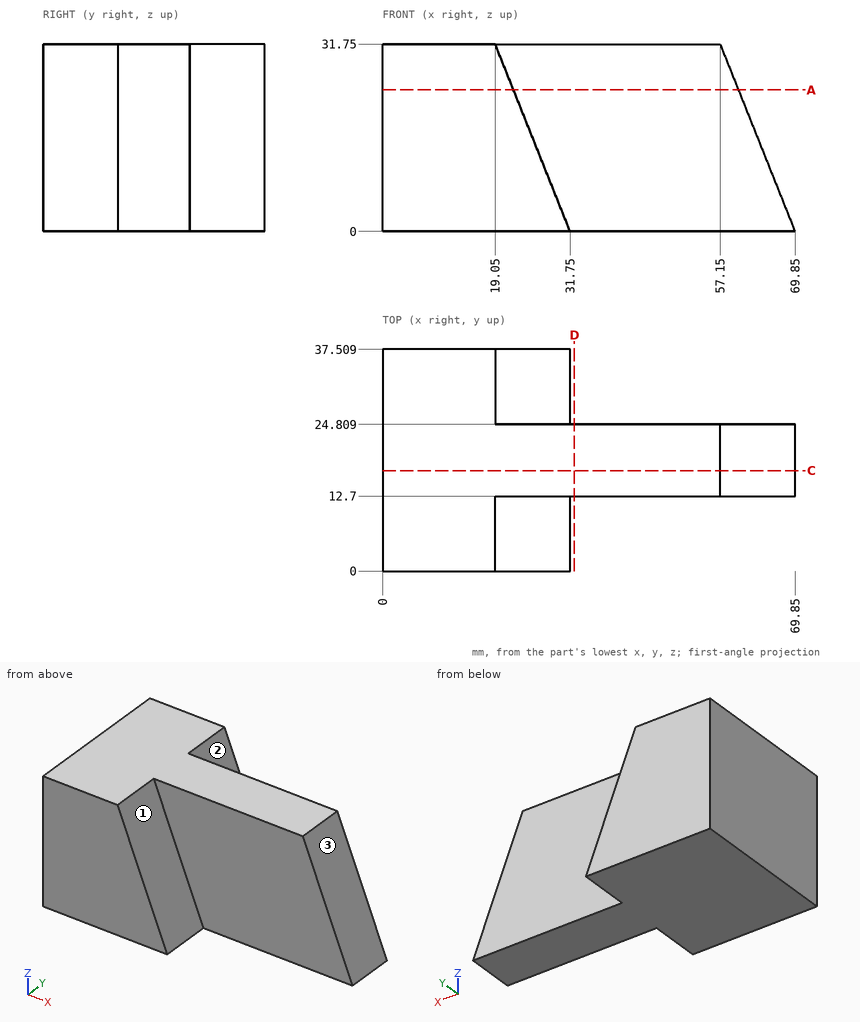
Geometry: see drawing. Coordinates: mm, zero at the bounding-box minimum. A direction names the side the tool comes from. Give positions to 0.01 mm unless a question says otherwise; leave off trailing zeros. Order: outer loops, then holes, each group sorted by start corner. A loop starts at its lowest first (then second) coordinate and runs counter-clockwise, first axis right, second up. Notation, with made-up numbers: (87, 42) - (105, 42) arc R30 ccw to (105, 68) - close; hole circle Ø6 at (37, 72.5). An arc over 180 degrees is marked (long way). One line per item, written item: value.
1. Reachability of the marked faces 1, 2 and 3 from +Z, -Z, +X, -X, +Y, -Y: full face, straight path, thin tool, end or side. Return the list, or none.
Determined:
face 1: +Z, +X, -Y
face 2: +Z, +X, +Y
face 3: +Z, +X, +Y, -Y
2. Line query: probe 1 along Y at (x, z) = (45.5, 10); probe 2 along X at (y, z) = (20.5, 9); probe 3 along X at (y, z) = (17, 15). Output: solid intervals per line, ascending.
Determined:
probe 1: 12.7 to 24.81
probe 2: 0 to 66.25
probe 3: 0 to 63.85
3. Cut plane A-A, the plane z = 24. Output: boundary loops of the cut face in (x, y).
Determined:
outline: (0, 0) - (22.15, 0) - (22.15, 12.7) - (60.25, 12.7) - (60.25, 24.81) - (22.15, 24.81) - (22.15, 37.51) - (0, 37.51) - close
4. Cut plane C-C, the plane y = 17. Output: boundary loops of the cut face in (x, z), and give its area (3 significant figures).
Determined:
outline: (0, 0) - (69.85, 0) - (57.15, 31.75) - (0, 31.75) - close
area: 2,020 mm2
5. Cut plane D-D, the plane x = 32.5. Output: boundary loops of the cut face in (y, z).
Determined:
outline: (12.7, 0) - (24.81, 0) - (24.81, 31.75) - (12.7, 31.75) - close
6. Pin query (flat end, axial travel): pin 1 Ø3 at (y, z) = (18.5, 21.5) entering from +X; pin 2 Ø10 at (y, z) = (31, 28) entering from -X; pin 3 Ø16 at (x, z) = (32, 22) entering from -Y; pin 4 Ø6 at (y, z) = (10.5, 20.5) entering from +X (1 decimal). Return the tip coordinate at first contact, or that it passes through.
Determined:
pin 1: x = 61.85
pin 2: x = 0
pin 3: y = 12.7
pin 4: x = 62.5
